For this review, take the finished solid that the model builds, in its own axes (mm). Face numbers are marked on the shaded views. A direction names the side the tool comes from. Coordinates: 2 decimals unless noted, no trailing zeros. Write each loop counter-clockwise with the first axis right and the second up, starting at its lowest first coordinate (ties: lowest second). Pieces come first, ordered by that corner, then holes. Notation, with made-up numbers: (-9.75, 41) -> (19.25, 41) arc R24 ccw to (19.25, 59) -> close; hole circle Ø6 at (37, -27). An arc over 180 degrees is marked (long way). One line per item, written item: value. Start each with the question number.
1) For probe 1 along Y at (x, z) = (0, 48); probe 2 along X at (y, z) = (0, 16); probe 3 along Y at (x, z) = (0, 10), list the stretches that pass through material, from the lowest coordinate up. Write a range as from..to.
2) Mouldability with a two-part tool opening along Y and no side actions: class the marked faces 3, 4 and 5 as released by +Y, released by -Y, zero draft, split by the parting line, or undercut.
3) Add section D-D (z = 5). State the section outline as (x, y) points (1 decimal).
4) Machinability: for the marked faces 1 and 2, which of the approach directions +Z, -Z, +X, -X, +Y, -Y give a long, thin tool a straight path to every point of the face, cutting with its end or side? Answer none if there is none.
5) Add section C-C (z = 24). State the section outline as (x, y) points, and give its area (3 significant figures).
6) Add section A-A (y = 0). State the section outline as (x, z) points, and give its area (3 significant figures).
7) For pin 1 Ø4 at (x, y) = (-7.5, 24) entering from -Z; pin 2 Ø10 at (x, z) = (3, 11.5) entering from +Y; pin 3 Ø3 at (x, y) = (-5, -0.5) entering from -Z, all flat-tipped, find the tip position at first contact; note any pin that passes through.
from build123d import *

# Parameters (mm, degrees)
F2_R     = 4.6355
F3_DEPTH = 13.97
F4_R     = 1.5875
F5_DEPTH = 20.32


with BuildPart() as f1:
    # F0 (on Front) → F1 (revolve)
    with BuildSketch(Plane.XZ):
        Polygon((0, 58.42), (0, 0), (35.56, 26.67), (35.56, 39.37), (12.7, 39.37), (12.7, 58.42), align=None)
    revolve(axis=Axis((0, 0, 29.21), (0, 0, -1)))

    # F2 (on face) → F3 (cut)
    with BuildSketch(Plane.XY.offset(58.42)):
        Circle(F2_R)
    extrude(amount=-F3_DEPTH, mode=Mode.SUBTRACT)

    # F4 (on Top) → F5 (cut)
    with BuildSketch(Plane.XY):
        Circle(F4_R)
    extrude(amount=F5_DEPTH, mode=Mode.SUBTRACT)


solid = f1.part
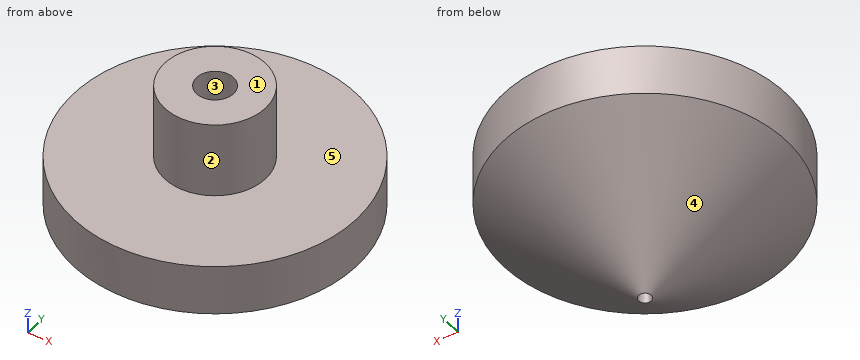
Numbers:
1. probe 1: -12.7..-4.64, 4.64..12.7
1. probe 2: -21.33..-1.59, 1.59..21.33
1. probe 3: -13.33..-1.59, 1.59..13.33
2. face 3: undercut
2. face 4: split by the parting line
2. face 5: zero draft
3. outline: circle Ø13.3 at (0, 0); hole circle Ø3.2 at (0, 0)
4. face 1: +Z, +X, -X, +Y, -Y
4. face 2: +Z
5. outline: circle Ø64 at (0, 0)
5. area: 3,220 mm²
6. outline: (-35.56, 26.67) -> (-1.59, 1.19) -> (-1.59, 20.32) -> (1.59, 20.32) -> (1.59, 1.19) -> (35.56, 26.67) -> (35.56, 39.37) -> (12.7, 39.37) -> (12.7, 58.42) -> (4.64, 58.42) -> (4.64, 44.45) -> (-4.64, 44.45) -> (-4.64, 58.42) -> (-12.7, 58.42) -> (-12.7, 39.37) -> (-35.56, 39.37) -> close
6. area: 2,140 mm²
7. pin 1: z = 17.36
7. pin 2: y = 21.82
7. pin 3: z = 2.64
